from build123d import *

# Parameters (mm, degrees)
EXTRUDE1_DEPTH = 12.7
FILLET1_R      = 2.54


with BuildPart() as part:
    # Sketch1 → Extrude1 (new body)
    with BuildSketch(Plane(origin=(0, 0, 0), x_dir=(1, 0, 0), z_dir=(0, 1, 0))):
        Polygon((-63.5, 0), (-83.917728463, 76.2), (-90.05135746, 74.556499064), (-68.372526374, -6.35), (0, -6.35), (0, 0), align=None)
        Polygon((63.5, 0), (0, 0), (0, -6.35), (68.372526374, -6.35), (90.05135746, 74.556499064), (83.917728463, 76.2), align=None)
    extrude(amount=EXTRUDE1_DEPTH)

    # Fillet1
    fillet1_edges = [part.edges().sort_by_distance(p)[0] for p in [
        (73.708864232, 12.7, -38.1),
        (0, 12.7, 0),
        (-73.708864232, 12.7, -38.1),
        (-73.708864232, 0, -38.1),
        (0, 0, 0),
        (73.708864232, 0, -38.1),
    ]]
    fillet(fillet1_edges, radius=FILLET1_R)


solid = part.part
Read the model definition and answer for the solid it produces. Units are mm, in the model's axes. A direction names the side the tool comes from. Round coordinates to 2 decimals unless told otherwise and drop trailing zeros. Write each loop counter-clockwise with the first axis right and the second up, starting at its lowest first coordinate (ties: lowest second). Pieces come first, ordered by that corner, then holes.
1. The part is cut by section B-B, the plane x = -26. Determine the outline of the cut face in (y, z).
2. Which of the six approach directions +Z, -Z, +X, -X, +Y, -Y give full straight-line access (tool end or side, diameter ignored) to faces 1 (the face through (1, 6, 0)), 2 (the face through (-74.303, 0.764, -37.518)), 3 (the face through (74.01, 11.94, -36.42)), 4 (the face through (-79.364, 6.261, -34.67))?
3. The part is cut by section A-A, the plane y = 5.75. Determine the outline of the cut face in (x, z), then the cut area to 3 significant figures.
4. Given pin 1 Ø1 at (y, z) = (6, -27.5) entering from +X; pin 2 Ø5 at (x, z) = (-71.5, -40.5) entering from -Y; pin 3 Ø1 at (x, y) = (-5, 9.5) entering from -Z, each flat-ended and moving along its own axis, determine where each tip first touches the part or whether it passes through.
5. Determine the mould class of faces 5 (the face through (-73.566, 6.297, -37.567)), 6 (the face through (79.06, 6.26, -33.54)), 7 (the face through (0, 0, 5)) for opening direction X: pulls with the +X half, pulls with the -X half, needs draft (parallel to the pull), parting line crosses it, or undercut.
6. Straight lines are drawn through the part: L1, parallel to X at y = 3, z = -7.5; L2, parallel to X at y = 11, z = -37.5; L3, parallel to Z at x = -29.5, y = 6. For each, find the intervals that lie inside material, in ascending order.
Values:
1. outline: (0, 2.54) arc R2.54 ccw to (2.54, 0) - (10.16, 0) arc R2.54 ccw to (12.7, 2.54) - (12.7, 6.35) - (0, 6.35) - close
2. face 1: -Z, +Y, -Y
2. face 2: -Z, -Y
2. face 3: -Z, +Y
2. face 4: +Z, -X, +Y, -Y
3. outline: (-90.05, -74.56) - (-83.92, -76.2) - (-63.5, 0) - (63.5, 0) - (83.92, -76.2) - (90.05, -74.56) - (68.37, 6.35) - (-68.37, 6.35) - close
3. area: 1,870 mm2
4. pin 1: stops at x = 77.58
4. pin 2: passes through
4. pin 3: stops at z = 0
5. face 5: undercut
5. face 6: pulls with the +X half
5. face 7: needs draft
6. L1: x = -72.08 to -65.51, 65.51 to 72.08
6. L2: x = -80.12 to -73.7, 73.7 to 80.12
6. L3: z = 0 to 6.35
